Can you work these out from the model? Positions are in its coordinate system, mm. A direction names the side the tool comes from. Round coordinates to 2 decimals unless told otherwise and drop trailing zeros. Order: outer loops, then holes, each group sorted by start corner. A loop starts at its lowest first (then second) coordinate and runs counter-clockwise, first axis right, second up.
Q1. If we section it at B-B (x = 61): Please give me the cut outline in (y, z).
Q2. If we section it at C-C (y = -16.5): Please give me the cut outline in (x, z).
Q3. If we section it at A-A (z = -5): Please give me the cut outline in (x, y).
Q4. If we section it at D-D (y = -9.5): Please give me the cut outline in (x, z).
Q5. If I drill on line 1 (X direction, y = -32.5, z = 6.5); line 2 (Y direction, x = 28, z = 2.5); line 3 (Y direction, x = 33.5, z = 22.5), over which ranges is the centre line in solid material (lowest first)?
Q6. We'd pull the mould along X, two halves only. Please class faces 5 (the face through (80, 0, 9)), 6 (the face through (2.85, -28.64, 12.54)), 7 (the face through (152, -29, -5)), 8 (the face through (112.5, -29.1, 4.3)): pulls with the +X half, pulls with the -X half, needs draft (parallel to the pull), parting line crosses it, or undercut.
Q7. For faces 1 (the face through (157, -29, 0)), 2 (the face through (18.5, -29.1, 4.3)), 3 (the face through (80, -29, 18)), 4 (the face through (5, -29, 0)), which set-ups out of +Z, -Z, +X, -X, +Y, -Y let a thin tool reach every point of the face, with its end or its side?
Q8. Will these pins go through, and if not, where does the flat tip stop? P1, Ø2.5, axis at y = -21, z = -5.5, coming from the +X side; P2, Ø5.5, axis at x = 6, y = -43.5, coming from the -Z side; P3, Ø11, axis at x = 107.5, y = -37.5, coming from the +Z side.
from build123d import *

# Parameters (mm, degrees)
F1_DEPTH = 58
F2_W     = 18
F2_H     = 11
F3_DEPTH = 163.001
F4_R     = 3
F6_DEPTH = 38.001


with BuildPart() as f1:
    # F0 (on Front) → F1 (new body)
    with BuildSketch(Plane.XZ):
        with BuildLine():
            Line((134, 29), (29, 29))
            ThreePointArc((29, 29), (8.493903, 20.506097), (0, 0))
            Line((0, 0), (11, 0))
            Line((11, 0), (11, -9))
            Line((11, -9), (152, -9))
            Line((152, -9), (152, 0))
            Line((152, 0), (163, 0))
            ThreePointArc((163, 0), (154.506097, 20.506097), (134, 29))
        make_face()
    extrude(amount=F1_DEPTH)

    # F2 (on Right) → F3 (cut, through all)
    with BuildSketch(Plane.YZ):
        with Locations((-38, 23.5)):
            Rectangle(F2_W, F2_H)
        with Locations((-20, 23.5)):
            Rectangle(F2_W, F2_H)
    extrude(amount=F3_DEPTH, mode=Mode.SUBTRACT)

    # F4
    f4_edges = [f1.edges().sort_by_distance(p)[0] for p in [
        (8.493903, -58, 20.506097),
        (81.5, -58, 29),
        (154.506097, -58, 20.506097),
        (8.493903, 0, 20.506097),
    ]]
    fillet(f4_edges, radius=F4_R)

    # F5 (on face) → F6 (cut, through all)
    with BuildSketch(Plane(origin=(0, 0, -9), x_dir=(1, 0, 0), z_dir=(0, 0, -1))):
        with BuildLine():
            ThreePointArc((138, 22.5), (142.596194, 24.403806), (144.5, 29))
            ThreePointArc((144.5, 29), (142.596194, 33.596194), (138, 35.5))
            ThreePointArc((138, 35.5), (131.5, 29), (138, 22.5))
        make_face()
        with BuildLine():
            ThreePointArc((138, 22.5), (131.5, 29), (138, 35.5))
            Line((138, 35.5), (119, 35.5))
            ThreePointArc((119, 35.5), (123.596194, 33.596194), (125.5, 29))
            ThreePointArc((125.5, 29), (123.596194, 24.403806), (119, 22.5))
            Line((119, 22.5), (138, 22.5))
        make_face()
        with BuildLine():
            ThreePointArc((125.5, 29), (123.596194, 33.596194), (119, 35.5))
            ThreePointArc((119, 35.5), (112.5, 29), (119, 22.5))
            ThreePointArc((119, 22.5), (123.596194, 24.403806), (125.5, 29))
        make_face()
        with BuildLine():
            ThreePointArc((25, 22.5), (29.596194, 24.403806), (31.5, 29))
            ThreePointArc((31.5, 29), (29.596194, 33.596194), (25, 35.5))
            ThreePointArc((25, 35.5), (18.5, 29), (25, 22.5))
        make_face()
        with BuildLine():
            ThreePointArc((25, 35.5), (29.596194, 33.596194), (31.5, 29))
            ThreePointArc((31.5, 29), (29.596194, 24.403806), (25, 22.5))
            Line((25, 22.5), (44, 22.5))
            ThreePointArc((44, 22.5), (37.5, 29), (44, 35.5))
            Line((44, 35.5), (25, 35.5))
        make_face()
        with BuildLine():
            ThreePointArc((50.5, 29), (48.596194, 33.596194), (44, 35.5))
            ThreePointArc((44, 35.5), (37.5, 29), (44, 22.5))
            ThreePointArc((44, 22.5), (48.596194, 24.403806), (50.5, 29))
        make_face()
    extrude(amount=-F6_DEPTH, mode=Mode.SUBTRACT)


solid = f1.part
Solution:
1. outline: (-58, -9) - (0, -9) - (0, 26) arc R3 ccw to (-3, 29) - (-11, 29) - (-11, 18) - (-47, 18) - (-47, 29) - (-55, 29) arc R3 ccw to (-58, 26) - close
2. outline: (0, 0) - (11, 0) - (11, -9) - (152, -9) - (152, 0) - (163, 0) arc R29 ccw to (156.74, 18) - (6.26, 18) arc R29 ccw to start
3. outline: (11, -58) - (152, -58) - (152, 0) - (11, 0) - close; hole (25, -35.5) - (44, -35.5) arc R6.5 ccw to (44, -22.5) - (25, -22.5) arc R6.5 ccw to start; hole (119, -35.5) - (138, -35.5) arc R6.5 ccw to (138, -22.5) - (119, -22.5) arc R6.5 ccw to start
4. outline: (0, 0) - (11, 0) - (11, -9) - (152, -9) - (152, 0) - (163, 0) arc R29 ccw to (134, 29) - (29, 29) arc R29 ccw to start
5. line 1: x = 0.74 to 19.52, 49.48 to 113.52, 143.48 to 162.26
5. line 2: y = -58 to -35.5, -22.5 to 0
5. line 3: y = -58 to -47, -11 to 0
6. face 5: needs draft
6. face 6: pulls with the -X half
6. face 7: pulls with the +X half
6. face 8: undercut
7. face 1: -Z, +X, +Y, -Y
7. face 2: +Z, -Z
7. face 3: +Z, +X, -X
7. face 4: -Z, -X, +Y, -Y
8. P1: stops at x = 152
8. P2: stops at z = 0
8. P3: stops at z = 18
